Can you work these out from the model? Positions are in its coordinate system, mm. Face numbers are marked on the shaded views. A direction names the side the tool comes from. Round coordinates to 2 decimals unless told otherwise and drop trailing zeros. Loops run counter-clockwise (first coordinate to the right, second up) from the corner with the lowest first, then second, coordinate; pieces in that order, holes last. Notation, with made-up numbers: (75.25, -40) -> (90.25, -40) arc R19 cw to (90.25, -31) -> close; hole circle Ø9 at (16, -2.75). An arc over 180 degrees is marked (long way). Write item = value, one per line.
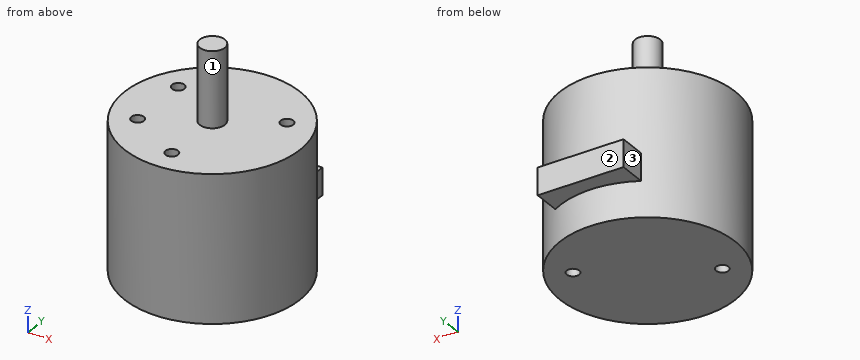
from build123d import *

# Parameters (mm, degrees)
SKETCH_1_R          = 21
EXTRUDE_1_DEPTH     = 35
SKETCH_2_R          = 3
EXTRUDE_2_DEPTH     = 18
EXTRUDE_4_DEPTH     = 6.5
SKETCH_7_R          = 1.5
CUT_EXTRUDE_1_DEPTH = 6.5
MM_PRESS_1_D        = 3
MM_PRESS_2_D        = 3


with BuildPart() as part:
    # 草图1 → 凸台-拉伸1 (new body)
    with BuildSketch(Plane.XY):
        Circle(SKETCH_1_R)
    extrude(amount=EXTRUDE_1_DEPTH)

    # 草图2 → 凸台-拉伸2 (add)
    with BuildSketch(Plane.XY.offset(35)):
        Circle(SKETCH_2_R)
    extrude(amount=EXTRUDE_2_DEPTH)

    # 草图6 → 凸台-拉伸4 (add)
    with BuildSketch(Plane(origin=(0, 0, 15), x_dir=(-1, 0, 0), z_dir=(0, 0, -1))):
        with BuildLine():
            Line((-10.25, 18.328597873), (-10.25, 24.828597873))
            Line((-10.25, 24.828597873), (10.25, 24.828597873))
            Line((10.25, 24.828597873), (10.25, 18.328597873))
            ThreePointArc((10.25, 18.328597873), (0, 21), (-10.25, 18.328597873))
        make_face()
    extrude(amount=EXTRUDE_4_DEPTH)

    # 草图7 → 切除-拉伸1 (cut)
    with BuildSketch(Plane.XY.offset(35)):
        with Locations((13, 7.5)):
            Circle(SKETCH_7_R)
        with Locations((0.002409407, -14.995836032)):
            Circle(SKETCH_7_R)
        with Locations((-12.98076078, 7.508325625)):
            Circle(SKETCH_7_R)
        with Locations((-13, -7.5)):
            Circle(SKETCH_7_R)
    extrude(amount=-CUT_EXTRUDE_1_DEPTH, mode=Mode.SUBTRACT)

    # 大小mm Press 暗销孔1 (through all)
    with Locations(Plane(origin=(19.777789767, 155.433675327, 28.5), x_dir=(0.242616345, -0.970122317, 0), z_dir=(0, 0, 1))):
        with Locations((141.869357239, -42.466412685)):
            Hole(MM_PRESS_1_D / 2)

    # 大小mm Press 暗销孔2 (through all)
    with Locations(Plane(origin=(19.777789767, 155.433675327, 28.5), x_dir=(0.242616345, -0.970122317, 0), z_dir=(0, 0, 1))):
        with Locations((150.113167025, -71.32883809)):
            Hole(MM_PRESS_2_D / 2)


solid = part.part
1. I need wall thicknesses on line 1 (Z direction, x = -13.5, y = 10); line 2 (X direction, y = 6.5, z = 30.5); line 3 (Y direction, x = 0, z = 4.5). Which ranges of each line are inside material? Lowest first, please. Write a range as [from, to].
Entries:
line_1 = [0, 35]
line_2 = [-19.97, -14.09], [-11.87, 11.88], [14.12, 19.97]
line_3 = [-21, 21]
2. I'm going to push flat-ended pins straight in: pin 1 (2 mm diameter, centred on y = -10, z = 19, fed in from +X); pin 2 (7 mm diameter, centred on x = 1, y = 23, fed in from +Z); pin 3 (1.8 mm diameter, centred on x = -12.98, y = 7.51, fed in from -Z); pin 4 (3 mm diameter, centred on y = -6, z = 19.5, fed in from +X). Where does each tip first touch, or does it pass through?
Entries:
pin_1 = 18.97
pin_2 = 35
pin_3 = 0
pin_4 = 20.51
3. Suppose I cut it at C-C, the plane y = -7.5. List the corners of the cut face in (x, z) for me.
Entries:
outline = (-19.62, 0) -> (-14.5, 0) -> (-14.5, 35) -> (-19.62, 35) -> close; (-11.5, 0) -> (19.62, 0) -> (19.62, 35) -> (-11.5, 35) -> close
4. Suppose I cut it at B-B, the plane x = 0. List the corners of the cut face in (y, z) for me, and give its area (3 significant figures).
Entries:
outline = (-21, 0) -> (21, 0) -> (21, 8.5) -> (24.83, 8.5) -> (24.83, 15) -> (21, 15) -> (21, 35) -> (3, 35) -> (3, 53) -> (-3, 53) -> (-3, 35) -> (-13.5, 35) -> (-13.5, 28.5) -> (-16.5, 28.5) -> (-16.5, 35) -> (-21, 35) -> close
area = 1,580 mm²
5. Suppose I cut it at A-A, the plane y = 0. List the corners of the cut face in (x, z) for me.
Entries:
outline = (-21, 0) -> (21, 0) -> (21, 35) -> (3, 35) -> (3, 53) -> (-3, 53) -> (-3, 35) -> (-21, 35) -> close
6. For the marked faces 1, 2 and 3, which set-ups out of +Z, -Z, +X, -X, +Y, -Y let a thin tool reach every point of the face, with its end or its side?
Entries:
face_1 = +Z
face_2 = +Z, -Z, +X, -X, +Y
face_3 = +Z, -Z, -X, +Y
7. Suppose I cut it at D-D, the plane z = 32. List the corners of the cut face in (x, y) for me.
Entries:
outline = circle Ø42 at (0, 0); hole circle Ø3 at (-13, -7.5); hole circle Ø3 at (-12.98, 7.51); hole circle Ø3 at (0, -15); hole circle Ø3 at (13, 7.5)
